Read the model definition and answer for the solid it produces. Units are mm, in the model's axes. A direction names the side the tool comes from. Round coordinates to 2 decimals unless told otherwise and drop trailing zeros. Write each loop counter-clockwise with the first axis right and the second up, starting at its lowest first coordinate (ties: lowest second). Pieces come first, ordered by that corner, then holes. Notation, with made-up numbers: (-18.75, -1.75) -> (25.25, -1.75) arc R30 ccw to (25.25, 28.25) -> close; hole circle Ø7 at (20, -16). An arc over 180 degrees is marked (long way). Return JSON: item names as keys, results as strings. Group by question number.
(1) Given pin 1 (2 mm diameter, centred on x = 5.5, z = 30.5, fed in from +Y); pin 2 (4 mm diameter, centred on x = 2, y = 8.5, fed in from -Z), each flat-ended and moving along its own axis, determine where each tip first touches the part or whether it passes through.
(2) Straight lines are drawn through the part: line 1 (Y direction, x = 7, z = 32.8); line 2 (X direction, y = 11, z = 24.5); line 3 (X direction, y = 8, z = 32.6). For each, find the intervals that lie inside material, in ascending order.
(3) For faces 1 (the flat face through (-20.383, 5.916, 29.43)), 2 (the flat face through (0, 5, 34.5)), 3 (the flat face through (20.383, 5.916, 29.43)), determine the directions among +Z, -Z, +X, -X, +Y, -Y from which every point of the face is accessible in a straight line to the end or side of a thin tool.
(4) A cutting plane is placed at D-D on z = 29. Give the vertices of the cut face in (x, y), then the cut area to 3 significant figures.
(5) A cutting plane is placed at B-B on x = -9. Give the vertices of the cut face in (y, z), then the cut area to 3 significant figures.
(6) A cutting plane is placed at A-A on z = 22. Give the vertices of the cut face in (x, y), then the cut area to 3 significant figures.
(7) The mould has two halves that part along X. Classify faces 4 (the flat face through (-25.617, 5, 23)), 5 (the cylindrical face through (-10.5, 8.07, 33.07)), 6 (the flat face through (25.617, 5, 23)), 7 (the cylindrical face through (8.43, 8.45, 32.96)): released by +X, released by -X, zero draft, split by the parting line, or undercut.
(8) A cutting plane is placed at C-C on y = 8. Give the vertices of the cut face in (x, z).
Autodesk Inventor part; units mm, degrees
ref_plane "YZ Plane" through (0, 0, 0) normal (1, 0, 0) x (0, 1, 0)
ref_plane "XZ Plane" through (0, 0, 0) normal (0, 1, 0) x (-1, 0, 0)
ref_plane "XY Plane" through (0, 0, 0) normal (0, 0, 1) x (1, 0, 0)
ref_plane "Plano de trabajo1" through (16, 0, 22.5) normal (0, 0, -1) x (-1, 0, 0)
sketch "Boceto2" plane through (16, 0, 22.5) normal (0, 0, -1) x (-1, 0, 0)
  line L0 (-6.5, 0) -> (0, 0)
  line L1 (0, 0) -> (32, 0)
  circle A0 centre (8, 8) radius 1.5
  circle A1 centre (24, 8) radius 1.5
  point P0 (16, 0)
  dimension "d15" = 3
  dimension "d16" = 3
extrude "Extrusión2" [suppressed]
ref_plane "Plano de trabajo2" through (0, 0, 0) normal (0, -1, 0) x (1, 0, 0)
sketch "Boceto4" plane through (0, 0, 0) normal (0, -1, 0) x (1, 0, 0)
  circle A0 centre (0, 0) radius 32.5
  arc A1 (28.2887, 16) -> (-28.2887, 16) centre (0, 0) ccw
  line L0 (0, 32.5) -> (0, 34.5)
  line L1 (0, 34.5) -> (-26.2329, 34.5)
  line L2 (-26.2329, 34.5) -> (30.7149, 34.5)
  line L3 (0, 0) -> (0, 20)
  arc A2 (28.2887, 16) -> (-28.2887, 16) centre (0, 0) ccw
  line L4 (0, 20) -> (50, 20)
  line L5 (50, 20) -> (-50, 20)
  line L6 (0, 34.5) -> (15, 34.5)
  line L7 (15, 34.5) -> (25.6174, 20)
  line L8 (0, 34.5) -> (-15, 34.5)
  line L9 (-15, 34.5) -> (-25.6174, 20)
  point P0 (-25.6174, 20)
  dimension "d19" = 2
  dimension "d20" = 20
  dimension "d21" = 50
  dimension "d22" = 100
  dimension "d23" = 15
  dimension "d24" = 15
extrude "Extrusión3" add sketch "Boceto4" against normal blind 12 contours A0 L0 L2 L7 | L9 L1 L0 A0
sketch "Boceto5" plane through (-15, 0, 34.5) normal (0, 0, 1) x (1, 0, 0)
  line L0 (30, 0) -> (30, 12)
  line L1 (30, 0) -> (30, 8)
  line L2 (30, 8) -> (22, 8)
  line L3 (22, 8) -> (6, 8)
  circle A0 centre (22, 8) radius 1.5
  circle A1 centre (6, 8) radius 1.5
  point P0 (15, 0)
  dimension "d27" = 8
  dimension "d28" = 8
  dimension "d29" = 16
  dimension "d30" = 3
  dimension "d31" = 3
extrude "Extrusión4" cut sketch "Boceto5" against normal blind 12
sketch "Boceto6" plane through (0, 0, 0) normal (0, -1, 0) x (1, 0, 0)
  circle A0 centre (0, 0) radius 32.5
  arc A1 (25.6174, 20) -> (-25.6174, 20) centre (0, 0) ccw
  line L0 (-15, 34.5) -> (15, 34.5)
  line L1 (25.6174, 20) -> (15, 34.5)
  line L2 (15, 34.5) -> (-15, 34.5)
  line L3 (-15, 34.5) -> (-25.6174, 20)
extrude "Extrusión5" add sketch "Boceto6" along normal blind 2 contours A0 L3 L0 L1
sketch "Boceto7" plane through (0, -2, 0) normal (0, -1, 0) x (1, 0, 0)
  line L0 (-25.6174, 20) -> (-15, 34.5)
  line L1 (-15, 34.5) -> (-25.6174, 34.5)
  line L2 (-25.6174, 34.5) -> (-25.6174, 20)
  line L3 (-25.6174, 20) -> (25.6174, 20)
  line L4 (25.6174, 20) -> (25.6174, 34.5)
  line L5 (25.6174, 20) -> (15, 34.5)
  line L6 (15, 34.5) -> (25.6174, 34.5)
  circle A0 centre (0, 0) radius 32.5
  line L7 (-15, 34.5) -> (15, 34.5)
extrude "Extrusión6" add sketch "Boceto7" along normal blind 8 contours L2 L1 L0 | A0 L3 | L0 L7 L5 A0 | L5 L6 L4 picked at (-1.7193, 25.9173)
sketch "Boceto8" plane through (-15, 12, 34.5) normal (0, 0, 1) x (1, 0, 0)
  line L0 (40.6174, -22) -> (-10.6174, -22)
  line L1 (-10.6174, -22) -> (-10.6174, -42.5)
  line L2 (-10.6174, -42.5) -> (39.7361, -42.5)
  line L3 (40.6174, -22) -> (40.6174, -42.5)
  line L4 (40.6174, -42.5) -> (39.7361, -42.5)
  line L5 (-10.6174, -22) -> (40.6174, -22)
  line L6 (40.6174, -14) -> (40.6174, -22)
  line L7 (-10.6174, -22) -> (40.6174, -22)
  line L8 (15, -22) -> (35.2, -22)
  line L9 (35.2, -22) -> (35.2, -42.5)
  line L10 (15, -22) -> (-5.2, -22)
  line L11 (-5.2, -22) -> (-5.2, -42.5)
  line L12 (-5.2, -42.5) -> (-5.2, -37.5)
  line L13 (-5.2, -22) -> (-5.2, -29)
  line L14 (-5.2, -29) -> (-10.6174, -29)
  line L15 (-5.2, -42.5) -> (-5.2, -36.5)
  line L16 (-5.2, -36.5) -> (-10.6174, -36.5)
  point P0 (15, -12)
  dimension "d38" = 20.5
  dimension "d39" = 20.5
  dimension "d40" = 20.2
  dimension "d41" = 20.2
  dimension "d43" = 7
  dimension "d44" = 6
extrude "Extrusión7" add sketch "Boceto8" against normal blind 14.5 contours L3 L4 L2 L9 L0 | L11 L14 L1 L0 | L2 L1 L16 L11
sketch "Boceto9" plane through (20.2, -30.5, 34.5) normal (0, -1, 0) x (1, 0, 0)
  line L0 (5.4174, -14.5) -> (5.4174, 0)
  line L1 (-45.8174, 0) -> (-45.8174, -14.5)
  line L2 (5.4174, 0) -> (-45.8174, 0)
  line L3 (-45.8174, 0) -> (-45.8174, -14.5)
  line L4 (-45.8174, -14.5) -> (5.4174, -14.5)
  line L5 (5.4174, 0) -> (-5.2, 0)
  line L6 (5.4174, -14.5) -> (5.4174, 0)
  point P0 (-20.2, -34.5)
extrude "Extrusión8" add sketch "Boceto9" along normal blind 5
sketch "Boceto10" plane through (0, -2, 0) normal (0, 1, 0) x (1, 0, 0)
  line L0 (-15, -34.5) -> (-25.6174, -34.5)
  line L1 (-15, -34.5) -> (-25.6174, -34.5)
  line L2 (-25.6174, -34.5) -> (-25.6174, -24.5)
  line L3 (-25.6174, -34.5) -> (-25.6174, -20)
  line L4 (-25.6174, -24.5) -> (-15, -34.5)
  line L5 (-25.6174, -20) -> (25.6174, -20)
  line L6 (-25.6174, -24.5) -> (-25.6174, -20)
  line L7 (-25.6174, -20) -> (-15, -34.5)
  line L8 (-15, -34.5) -> (-25.6174, -20)
  arc A0 (-25.6174, -20) -> (25.6174, -20) centre (0, 0) ccw
  line L9 (0, -32.5) -> (0, -25.3096)
  line L10 (15, -34.5) -> (25.6174, -34.5)
  line L11 (25.6174, -34.5) -> (25.6174, -24.5)
  line L12 (25.6174, -34.5) -> (25.6174, -20)
  line L13 (25.6174, -24.5) -> (15, -34.5)
  line L14 (25.6174, -20) -> (15, -34.5)
  dimension "d49" = 10
extrude "Extrusión9" add sketch "Boceto10" along normal blind 14 contours L12 L13 L14 | L4 L3 L7
sketch "Boceto11" plane through (-25.6174, -17, 34.5) normal (0, 0, 1) x (1, 0, 0)
  line L0 (45.8174, 7) -> (45.8174, -13.5)
  line L1 (45.8174, -13.5) -> (45.8174, 7)
  line L2 (45.8174, 7) -> (45.8174, -3.25)
  point P0 (25.6174, 17)
chamfer "Chaflán1" distance 2 angle 45 2 edges at (20.3087, -2, 29.5) (-20.3087, -2, 29.5)
sketch "Boceto12" plane through (0, -2, 0) normal (0, 1, 0) x (1, 0, 0)
  line L0 (40.0402, -40.6139) -> (-53.4832, -40.6139)
  line L1 (-53.4832, -40.6139) -> (-53.4832, 20.2117)
  line L2 (-53.4832, 20.2117) -> (40.0402, 20.2117)
  line L3 (40.0402, 20.2117) -> (40.0402, -40.6139)
  point P0 (0, 0)
extrude "Extrusión10" cut sketch "Boceto12" against normal blind 100
sketch "Boceto14" plane through (-15, 12, 34.5) normal (0, 0, 1) x (1, 0, 0)
  line L0 (-2.917, -14) -> (32.917, -14)
  line L1 (40.6174, -14) -> (-10.6174, -14)
  line L2 (15, -14) -> (7.5, -14)
  line L3 (7.5, -14) -> (7.5, -34.2047)
  line L4 (7.5, -14) -> (17.5, -14)
  line L5 (17.5, -14) -> (17.5, -67.4)
  line L6 (17.5, -67.4) -> (-2.5, -67.4)
  line L7 (-2.917, -14) -> (0, -12)
  line L8 (7.5, -14) -> (-2.5, -14)
  line L9 (-2.5, -14) -> (-2.5, -67.4)
  line L10 (-2.5, -14) -> (-2.5, -16.6)
  line L11 (-2.5, -16.6) -> (2.55, -16.6)
  line L12 (2.55, -16.6) -> (12.45, -16.6)
  line L13 (12.45, -16.6) -> (17.5, -16.6)
  circle A0 centre (12.45, -16.6) radius 2.2
  circle A1 centre (0.025, -16.6) radius 2.2
  line L14 (17.5, -67.4) -> (17.5, -64.8)
  line L15 (17.5, -64.8) -> (12.45, -64.8)
  line L16 (12.45, -64.8) -> (2.55, -64.8)
  line L17 (2.55, -64.8) -> (-2.5, -64.8)
  circle A2 centre (12.45, -64.8) radius 2.2
  circle A3 centre (2.55, -64.8) radius 2.2
  point P0 (15, -12)
  dimension "d59" = 10
  dimension "d60" = 53.4
  dimension "d61" = 20
  dimension "d68" = 2.6
  dimension "d69" = 5.05
  dimension "d70" = 9.9
  dimension "d71" = 5.05
  dimension "d72" = 4.4
  dimension "d73" = 4.4
  dimension "d74" = 2.6
  dimension "d75" = 5.05
  dimension "d76" = 9.9
  dimension "d77" = 5.05
  dimension "d78" = 4.4
  dimension "d79" = 4.4
properties part number "to_wily"
Checks:
{
 "1": {"pin 1": "passes through", "pin 2": "stops at z = 32.25"},
 "2": {"line 1": "y = -2 to 6.5, 9.5 to 12", "line 2": "x = -25.62 to -21.35, 21.35 to 25.62", "line 3": "x = -17.02 to -10.5, -7.5 to 5.5, 8.5 to 17.02"},
 "3": {"face 1": "+Z, -X, +Y", "face 2": "+Z, +X, -X, +Y, -Y", "face 3": "+Z, +X, +Y"},
 "4": {"outline": "(-23.76, -2) -> (-14.67, -2) -> (-14.67, 12) -> (-20.84, 12) -> (-20.84, 0) -> close; (14.67, -2) -> (23.76, -2) -> (20.84, 0) -> (20.84, 12) -> (14.67, 12) -> close", "area": "179 mm^2"},
 "5": {"outline": "(-2, 31.23) -> (6.5, 31.23) -> (6.5, 34.5) -> (-2, 34.5) -> close; (9.5, 31.23) -> (12, 31.23) -> (12, 34.5) -> (9.5, 34.5) -> close", "area": "36.0 mm^2"},
 "6": {"outline": "(-25.62, -2) -> (-23.92, -2) -> (-23.92, 12) -> (-25.62, 12) -> close; (23.92, -2) -> (25.62, -2) -> (25.62, 12) -> (23.92, 12) -> close", "area": "47.5 mm^2"},
 "7": {"face 4": "released by -X", "face 5": "undercut", "face 6": "released by +X", "face 7": "undercut"},
 "8": {"outline": "(-25.62, 20) arc R32.5 cw to (-10.5, 30.76) -> (-10.5, 34.5) -> (-15, 34.5) -> (-25.62, 24.5) -> close; (-7.5, 31.62) arc R32.5 cw to (5.5, 32.03) -> (5.5, 34.5) -> (-7.5, 34.5) -> close; (8.5, 31.37) arc R32.5 cw to (25.62, 20) -> (25.62, 24.5) -> (15, 34.5) -> (8.5, 34.5) -> close"}
}
